Build history of the part. All positions in model axes, mm. Give positions to 0.01 mm unless a question says otherwise; leave off trailing zeros. Loops run counter-clockwise (first coordinate to the right, second up) from the corner with the lowest first, then second, coordinate; pieces in that order, holes last.
1) Flat gauge pins, fed straight in: P1, Ø6, axis at x = 39, y = -48.5, coming from the +Z side; P2, Ø1.5, axis at y = -29, z = 3.5, coming from the -X side; P3, Ø2.5, axis at y = -19, z = 3.5, coming from the -X side; P4, Ø2.5, axis at y = -66, z = 2.5, coming from the -X side. Where does each tip first touch, or does it go through?
2) Band-saw the part on B-B on y = -20. List the corners of the cut face in (x, z).
3) Wall check: line 1 (Y direction, x = 22, z = 2.6); line 2 (Y direction, x = 20.5, z = 1.55); line 3 (X direction, y = -63, z = 0.2) (3 decimals). Give the ranges that are in metal, low to high.
4) Band-saw the part on A-A on x = 36.5. List the corners of the cut face in (y, z).
5) Band-saw the part on D-D on y = 0.5. List the corners of the cut face in (x, z), then the cut area to 3 significant figures.
6) Band-saw the part on C-C on z = 3.2. State how many separate pieces and enclosed holes the cut face has, then the cut area to 3 significant figures.
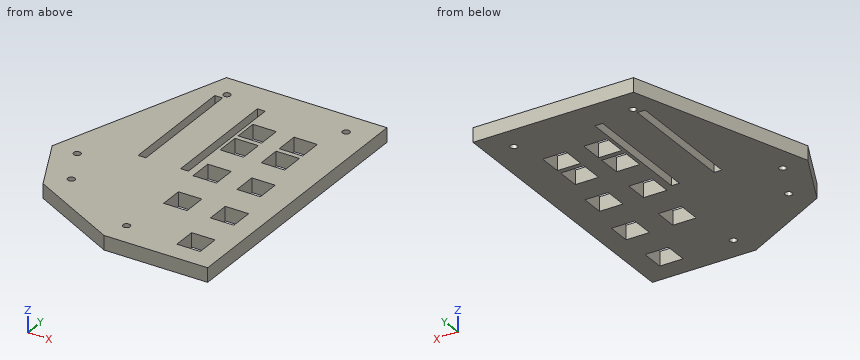
```python
from build123d import *

# Parameters (mm, degrees)
BOSS_EXTRUDE1_DEPTH = 5.08
SKETCH5_W           = 8.382
SKETCH5_H           = 8.382
SKETCH5_W_2         = 2.794
SKETCH5_H_2         = 43.434
CUT_EXTRUDE1_DEPTH  = 6.08
SKETCH7_R           = 1.27
CUT_EXTRUDE3_DEPTH  = 6.08


with BuildPart() as part:
    # Sketch1 → Boss-Extrude1 (new body)
    with BuildSketch(Plane.XY):
        Polygon((-4.120444444, 6.35), (53.34, 6.35), (53.34, -95.25), (16.22499019, -95.25), (-16.356614113, -78.274710363), (-26.416, -57.15), align=None)
    extrude(amount=BOSS_EXTRUDE1_DEPTH)

    # Sketch5 → Cut-Extrude1 (cut, through all)
    with BuildSketch(Plane(origin=(0, 0, 0), x_dir=(-1, 0, 0), z_dir=(0, 0, -1))):
        with Locations((-36.83, -17.78)):
            Rectangle(SKETCH5_W, SKETCH5_H)
        with Locations((-39.37, -45.72)):
            Rectangle(SKETCH5_W, SKETCH5_H)
        with Locations((-36.83, -27.94)):
            Rectangle(SKETCH5_W, SKETCH5_H)
        with Locations((-41.91, -64.77)):
            Rectangle(SKETCH5_W, SKETCH5_H)
        with Locations((-41.91, -83.82)):
            Rectangle(SKETCH5_W, SKETCH5_H)
        with Locations((-22.098, -17.78)):
            Rectangle(SKETCH5_W, SKETCH5_H)
        with Locations((-22.098, -27.94)):
            Rectangle(SKETCH5_W, SKETCH5_H)
        with Locations((-23.622, -45.72)):
            Rectangle(SKETCH5_W, SKETCH5_H)
        with Locations((-25.146, -64.77)):
            Rectangle(SKETCH5_W, SKETCH5_H)
        with Locations((-15.367, -26.543)):
            Rectangle(SKETCH5_W_2, SKETCH5_H_2)
        with Locations((-0.127, -26.543)):
            Rectangle(SKETCH5_W_2, SKETCH5_H_2)
    extrude(amount=-CUT_EXTRUDE1_DEPTH, mode=Mode.SUBTRACT)

    # Sketch7 → Cut-Extrude3 (cut, through all)
    with BuildSketch(Plane.XY.offset(5.08)):
        with Locations((44.2976, -2.4892)):
            Circle(SKETCH7_R)
        with Locations((1.6002, -2.4384)):
            Circle(SKETCH7_R)
        with Locations((-17.4498, -57.15)):
            Circle(SKETCH7_R)
        with Locations((-10.5918, -71.3486)):
            Circle(SKETCH7_R)
        with Locations((18.796, -86.5378)):
            Circle(SKETCH7_R)
    extrude(amount=-CUT_EXTRUDE3_DEPTH, mode=Mode.SUBTRACT)


solid = part.part
```
Findings below:
1. P1: stops at z = 5.08
1. P2: stops at x = -16.8
1. P3: stops at x = -13.46
1. P4: stops at x = -22.8
2. outline: (-13.37, 0) - (-1.27, 0) - (-1.27, 5.08) - (-13.37, 5.08) - close; (1.52, 0) - (13.97, 0) - (13.97, 5.08) - (1.52, 5.08) - close; (16.76, 0) - (17.91, 0) - (17.91, 5.08) - (16.76, 5.08) - close; (26.29, 0) - (32.64, 0) - (32.64, 5.08) - (26.29, 5.08) - close; (41.02, 0) - (53.34, 0) - (53.34, 5.08) - (41.02, 5.08) - close
3. line 1: y = -95.25 to -68.96, -60.58 to -49.91, -41.53 to -32.13, -23.75 to -21.97, -13.59 to 6.35
3. line 2: y = -95.25 to -49.91, -41.53 to -32.13, -23.75 to -21.97, -13.59 to 6.35
3. line 3: x = -23.63 to 20.955, 29.337 to 37.719, 46.101 to 53.34
4. outline: (-95.25, 0) - (-49.91, 0) - (-49.91, 5.08) - (-95.25, 5.08) - close; (-41.53, 0) - (-32.13, 0) - (-32.13, 5.08) - (-41.53, 5.08) - close; (-23.75, 0) - (-21.97, 0) - (-21.97, 5.08) - (-23.75, 5.08) - close; (-13.59, 0) - (6.35, 0) - (6.35, 5.08) - (-13.59, 5.08) - close
5. outline: (-6.17, 0) - (53.34, 0) - (53.34, 5.08) - (-6.17, 5.08) - close
5. area: 302 mm2
6. separate pieces: 1
6. enclosed holes: 16
6. area: 5,940 mm2
